Input: part model. Units: mm. Frame: model coordinates. Face numbers are marked on the shaded views. A direction names the side the tool comes from. Round coordinates to 2 decimals unless told otherwise and drop trailing zeros. Order: outer loops, then holes, each group sorted by start corner. A loop starts at its lowest first (then second) coordinate and runs counter-clockwise, first axis right, second up.
Item 1: First-contact query: pin 1 (6.5 mm diameter, centred on x = -49.45, y = -18.55, fed in from +Z). Flat tip, straight axial feed; report the tip coordinate or a pass-through.
Item 2: Reachability of the marked faces 1 and 2 from +Z, -Z, +X, -X, +Y, -Y: full face, straight path, thin tool, end or side. Return the list, or none.
Item 3: Cut plane B-B on y = -34. Output: boundary loops of the cut face in (x, z), then the cut area to 3 significant figures.
Item 4: Line query: L1, parallel to Y at x = 17.5, z = 18.25; L2, parallel to Z at x = -12.5, y = -51; L3, parallel to X at y = 17.5, z = 21.5. Output: solid intervals per line, ascending.
Item 5: Cut plane A-A on z = 3.5. Output: boundary loops of the cut face in (x, y).
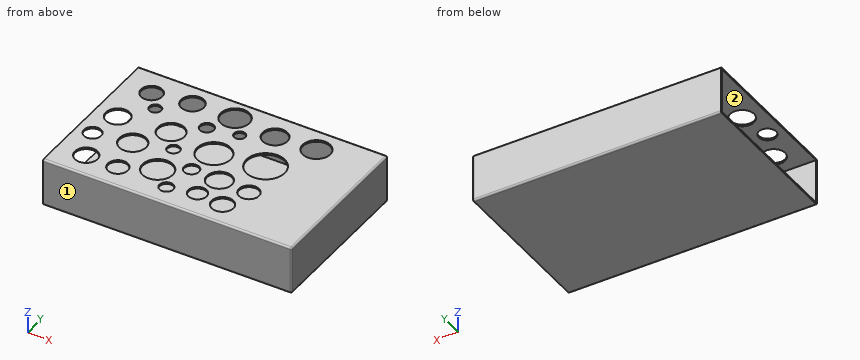
```python
from build123d import *

# Parameters (mm, degrees)
SKETCH001_W    = 139
SKETCH001_H    = 87
PAD_DEPTH      = 25
THICKNESS_T    = 1
SKETCH002_R    = 5.947053
SKETCH002_R_2  = 6.391543
SKETCH002_R_3  = 7.479707
SKETCH002_R_4  = 6.690044
SKETCH002_R_5  = 7.551468
SKETCH002_R_6  = 6.341994
SKETCH002_R_7  = 8.509486
SKETCH002_R_8  = 9.409582
SKETCH002_R_9  = 8.069876
SKETCH002_R_10 = 7.030828
SKETCH002_R_11 = 5.146618
SKETCH002_R_12 = 6.982672
SKETCH002_R_13 = 7.752117
SKETCH002_R_14 = 10.787845
SKETCH002_R_15 = 5.65876
SKETCH002_R_16 = 3.93116
SKETCH002_R_17 = 3.377122
SKETCH002_R_18 = 5.622868
SKETCH002_R_19 = 3.905324
SKETCH002_R_20 = 4.228889
SKETCH002_R_21 = 3.528588
SKETCH002_R_22 = 3.16034
SKETCH002_R_23 = 6.106178
SKETCH002_R_24 = 4.85306
POCKET_DEPTH   = 5


with BuildPart() as part:
    # Sketch001 → Pad (new body)
    with BuildSketch(Plane.XY):
        with Locations((-29.136072, -13.994338)):
            Rectangle(SKETCH001_W, SKETCH001_H)
    extrude(amount=PAD_DEPTH)

    # Thickness
    thickness_openings = [part.faces().sort_by_distance(p)[0] for p in [
        (-98.636072, -13.994338, 12.5),
    ]]
    offset(amount=THICKNESS_T, openings=thickness_openings)

    # Sketch002 (on Face14 of Thickness) → Pocket (cut)
    with BuildSketch(Plane.XY.offset(26)):
        with Locations((-82.334571, 15.216334)):
            Circle(SKETCH002_R)
        with Locations((-61.021297, 18.021215)):
            Circle(SKETCH002_R_2)
        with Locations((-57.73288, -7.189993)):
            Circle(SKETCH002_R_3)
        with Locations((-86.232513, -9.656311)):
            Circle(SKETCH002_R_4)
        with Locations((-68.946266, -24.274019)):
            Circle(SKETCH002_R_5)
        with Locations((-82.723099, -44.663734)):
            Circle(SKETCH002_R_6)
        with Locations((-47.27071, -36.765015)):
            Circle(SKETCH002_R_7)
        with Locations((-30.922209, -11.599332)):
            Circle(SKETCH002_R_8)
        with Locations((-37.351395, 18.526012)):
            Circle(SKETCH002_R_9)
        with Locations((-17.329054, -28.866299)):
            Circle(SKETCH002_R_10)
        with Locations((-20.819183, -43.377895)):
            Circle(SKETCH002_R_11)
        with Locations((-12.920469, 15.403262)):
            Circle(SKETCH002_R_12)
        with Locations((9.489837, 16.872791)):
            Circle(SKETCH002_R_13)
        with Locations((-4.286991, -7.558129)):
            Circle(SKETCH002_R_14)
        with Locations((0, -29.968445)):
            Circle(SKETCH002_R_15)
        with Locations((-44.858665, 4.777251)):
            Circle(SKETCH002_R_16)
        with Locations((-74.249245, 5.328322)):
            Circle(SKETCH002_R_17)
        with Locations((-64.697304, -45.003048)):
            Circle(SKETCH002_R_18)
        with Locations((-36.225178, -46.839958)):
            Circle(SKETCH002_R_19)
        with Locations((-33.469814, -28.103462)):
            Circle(SKETCH002_R_20)
        with Locations((-49.450947, -18.551527)):
            Circle(SKETCH002_R_21)
        with Locations((-28.142773, 7.716309)):
            Circle(SKETCH002_R_22)
        with Locations((-5.732456, -45.003048)):
            Circle(SKETCH002_R_23)
        with Locations((-89.679298, -27.368698)):
            Circle(SKETCH002_R_24)
    extrude(amount=-POCKET_DEPTH, mode=Mode.SUBTRACT)


solid = part.part
```
From the geometry:
1. pin 1: stops at z = 0
2. face 1: +Z, -Z, +X, -X, -Y
2. face 2: -X
3. outline: (-98.64, -1) - (40.36, -1) arc R1 ccw to (41.36, 0) - (41.36, 25) arc R1 ccw to (40.36, 26) - (3.97, 26) - (3.97, 25) - (40.36, 25) - (40.36, 0) - (-98.64, 0) - close; (-98.64, 25) - (-55.32, 25) - (-55.32, 26) - (-98.64, 26) - close; (-39.22, 25) - (-22.13, 25) - (-22.13, 26) - (-39.22, 26) - close; (-12.53, 25) - (-3.97, 25) - (-3.97, 26) - (-12.53, 26) - close
3. area: 271 mm2
4. L1: y = -58.49 to -57.49, 29.51 to 30.51
4. L2: z = -1 to 0, 25 to 26
4. L3: x = 40.36 to 41.36
5. outline: (-98.64, -58.49) - (40.36, -58.49) arc R1 ccw to (41.36, -57.49) - (41.36, 29.51) arc R1 ccw to (40.36, 30.51) - (-98.64, 30.51) - (-98.64, 29.51) - (40.36, 29.51) - (40.36, -57.49) - (-98.64, -57.49) - close
